```python
from build123d import *

# Parameters (mm, degrees)
SKETCH_W     = 5
SKETCH_H     = 2.4
PAD_DEPTH    = 4.5
SKETCH001_W  = 4.6
SKETCH001_H  = 2
PAD001_DEPTH = 1
SKETCH002_W  = 5
SKETCH002_H  = 2.4
PAD002_DEPTH = 1
FILLET_R     = 0.1
FILLET001_R  = 0.1
FILLET002_R  = 0.1
SKETCH003_W  = 4.2
SKETCH003_H  = 1.6
POCKET_DEPTH = 6


with BuildPart() as part:
    # Sketch → Pad (new body)
    with BuildSketch(Plane.XZ):
        Rectangle(SKETCH_W, SKETCH_H)
    extrude(amount=-PAD_DEPTH)

    # Sketch001 (on Face6 of Pad) → Pad001 (join)
    with BuildSketch(Plane(origin=(0, 4.5, 0), x_dir=(1, 0, 0), z_dir=(0, 1, 0))):
        Rectangle(SKETCH001_W, SKETCH001_H)
    extrude(amount=PAD001_DEPTH)

    # Sketch002 (on Face11 of Pad001) → Pad002 (join)
    with BuildSketch(Plane(origin=(0, 5.5, 0), x_dir=(1, 0, 0), z_dir=(0, 1, 0))):
        Rectangle(SKETCH002_W, SKETCH002_H)
    extrude(amount=PAD002_DEPTH)

    # Fillet
    fillet_edges = [part.edges().sort_by_distance(p)[0] for p in [
        (2.5, 2.25, 1.2),
        (-2.5, 2.25, 1.2),
        (-2.5, 6, 1.2),
        (2.5, 6, 1.2),
        (2.5, 6, -1.2),
        (2.5, 2.25, -1.2),
        (-2.3, 5, 1),
        (2.3, 5, 1),
        (2.3, 5, -1),
        (-2.5, 2.25, -1.2),
        (-2.5, 6, -1.2),
        (-2.3, 5, -1),
    ]]
    fillet(fillet_edges, radius=FILLET_R)

    # Fillet001
    fillet001_edges = [part.edges().sort_by_distance(p)[0] for p in [
        (0, 6.5, -1.2),
        (2.5, 6.5, 0),
        (0, 6.5, 1.2),
        (-2.5, 6.5, 0),
    ]]
    fillet(fillet001_edges, radius=FILLET001_R)

    # Fillet002
    fillet002_edges = [part.edges().sort_by_distance(p)[0] for p in [
        (0, 5.5, -1.2),
        (0, 4.5, -1.2),
        (-2.5, 4.5, 0),
        (-2.5, 5.5, 0),
        (0, 4.5, 1.2),
        (2.5, 4.5, 0),
        (0, 5.5, 1.2),
        (2.5, 5.5, 0),
    ]]
    fillet(fillet002_edges, radius=FILLET002_R)

    # Sketch003 (on Face49 of Fillet002) → Pocket (cut)
    with BuildSketch(Plane.XZ):
        Rectangle(SKETCH003_W, SKETCH003_H)
    extrude(amount=-POCKET_DEPTH, mode=Mode.SUBTRACT)


solid = part.part
```
For this review, take the finished solid that the model builds, in its own axes (mm). A direction names the side the tool comes from. Give positions to 0.01 mm unless a question says otherwise; leave off trailing zeros. Loops run counter-clockwise (first coordinate to the right, second up) from the corner with the lowest first, then second, coordinate; pieces in that order, holes last. Notation, with made-up numbers: M -35.5,60.25 L -25.5,60.25 A19 ccw -25.5,94.25 Z; hole C 68.25,34.25 d7. An arc over 180 degrees is marked long. One line per item, written item: value. Start each with the question number.
Q1. Draft analysis for pull direction X (two halves, no side actions). For faces 4 (the face through (0, 6, 0)), 5 (the face through (2.5, 2, 0)), 6 (the face through (-2.1, 3, 0)), 7 (the face through (-2.5, 6, 0)), state which applies: released by +X, released by -X, zero draft, split by the parting line, or undercut.
Q2. Add section B-B (z = -0.25). Give the boundary of the cut face in (x, y), and give its area (3 significant figures).
Q3. Add section A-A (y = 5.25). Give the boundary of the cut face in (x, z).
Q4. For L1, parallel to Z at x = 1.7, y = 2; L2, parallel to Z at x = 0.65, y = 4.75; L3, parallel to X at y = 4, z = 0.5, list the stretches that pass through material, from the lowest coordinate up.
Q5. Machinability: for faces 1 (the face through (0, 3, -0.8)), 2 (the face through (2.3, 5, 0)), 3 (the face through (-2.3, 5, 0)), which of the approach directions +Z, -Z, +X, -X, +Y, -Y give a long, thin tool a straight path to every point of the face, cutting with its end or side? Answer none if there is none.
Q6. Add section C-C (x = 1.85). Give the boundary of the cut face in (y, z).
Q7. Add section D-D (y = 2.75). Give the boundary of the cut face in (x, z).
Q8. Clearance check with a flat-ended pin moving along its axis: pin 1 Ø0.8 at (y, z) = (5, 0) entering from +X. State where the tip first meets the part, or that it passes through.
Reply:
1. face 4: undercut
1. face 5: released by +X
1. face 6: undercut
1. face 7: released by -X
2. outline: M -2.5,0 L -2.1,0 L -2.1,6 L 2.1,6 L 2.1,0 L 2.5,0 L 2.5,4.4 A0.1 ccw 2.4,4.5 L 2.3,4.5 L 2.3,5.5 L 2.4,5.5 A0.1 ccw 2.5,5.6 L 2.5,6.4 A0.1 ccw 2.4,6.5 L -2.4,6.5 A0.1 ccw -2.5,6.4 L -2.5,5.6 A0.1 ccw -2.4,5.5 L -2.3,5.5 L -2.3,4.5 L -2.4,4.5 A0.1 ccw -2.5,4.4 Z
2. area: 6.89 mm²
3. outline: M -2.3,-0.9 A0.1 ccw -2.2,-1 L 2.2,-1 A0.1 ccw 2.3,-0.9 L 2.3,0.9 A0.1 ccw 2.2,1 L -2.2,1 A0.1 ccw -2.3,0.9 Z; hole M -2.1,-0.8 L 2.1,-0.8 L 2.1,0.8 L -2.1,0.8 Z
4. L1: -1.2 to -0.8, 0.8 to 1.2
4. L2: -1 to -0.8, 0.8 to 1
4. L3: -2.5 to -2.1, 2.1 to 2.5
5. face 1: -Y
5. face 2: +Z, -Z, +X
5. face 3: +Z, -Z, -X
6. outline: M 0,-1.2 L 4.4,-1.2 A0.1 ccw 4.5,-1.1 L 4.5,-1 L 5.5,-1 L 5.5,-1.1 A0.1 ccw 5.6,-1.2 L 6.4,-1.2 A0.1 ccw 6.5,-1.1 L 6.5,1.1 A0.1 ccw 6.4,1.2 L 5.6,1.2 A0.1 ccw 5.5,1.1 L 5.5,1 L 4.5,1 L 4.5,1.1 A0.1 ccw 4.4,1.2 L 0,1.2 L 0,0.8 L 6,0.8 L 6,-0.8 L 0,-0.8 Z
7. outline: M -2.5,-1.1 A0.1 ccw -2.4,-1.2 L 2.4,-1.2 A0.1 ccw 2.5,-1.1 L 2.5,1.1 A0.1 ccw 2.4,1.2 L -2.4,1.2 A0.1 ccw -2.5,1.1 Z; hole M -2.1,-0.8 L 2.1,-0.8 L 2.1,0.8 L -2.1,0.8 Z
8. pin 1: x = 2.3
